```python
from build123d import *

# Parameters (mm, degrees)
BASE_FLANGE1_DEPTH             = 762
HOLE1_OUTLINE_R                = 7.14375
HOLE1_DEPTH                    = 1.4986
LPATTERN1_COUNT                = 10
LPATTERN1_PITCH                = 139.7
F_5_16_0_3125_DIAMETER_HOLE1_D = 7.9375
LPATTERN2_COUNT                = 10
LPATTERN2_PITCH                = 139.7


# Read off the part's stored shape, not the designer's step: Hole1
# Sheet-metal steps are written as plain solids
with BuildPart() as part:
    # Sketch1 → Base-Flange1 (new, symmetric)
    with BuildSketch(Plane.XY):
        with BuildLine():
            Line((82.55, 50.8), (82.55, 3.0861))
            ThreePointArc((82.55, 3.0861), (81.646102237, 0.903897763), (79.4639, 0))
            Line((79.4639, 0), (-79.4639, 0))
            ThreePointArc((-79.4639, 0), (-81.646102237, 0.903897763), (-82.55, 3.0861))
            Line((-82.55, 3.0861), (-82.55, 50.8))
            Line((-82.55, 50.8), (-81.0514, 50.8))
            Line((-81.0514, 50.8), (-81.0514, 3.0861))
            ThreePointArc((-81.0514, 3.0861), (-80.586432015, 1.963567985), (-79.4639, 1.4986))
            Line((-79.4639, 1.4986), (79.4639, 1.4986))
            ThreePointArc((79.4639, 1.4986), (80.586432015, 1.963567985), (81.0514, 3.0861))
            Line((81.0514, 3.0861), (81.0514, 50.8))
            Line((81.0514, 50.8), (82.55, 50.8))
        make_face()
    extrude(amount=BASE_FLANGE1_DEPTH, both=True)

    # Hole1 outline → Hole1 (cut)
    with BuildSketch(Plane(origin=(0, 0, 0), x_dir=(1, 0, 0), z_dir=(0, 1, 0))):
        with Locations((0, 628.65)):
            Circle(HOLE1_OUTLINE_R)
    hole1 = extrude(amount=HOLE1_DEPTH, mode=Mode.SUBTRACT)

    # LPattern1: Hole1 ×10
    with Locations(*[(0, 0, i * LPATTERN1_PITCH) for i in range(1, LPATTERN1_COUNT)]):
        add(hole1, mode=Mode.SUBTRACT)

    # 5/16 (0.3125) Diameter Hole1 (through all)
    with Locations(Plane(origin=(0, 0, 0), x_dir=(-1, 0, 0), z_dir=(0, -1, 0))):
        with Locations((0, 660.4), (0, 596.9)):
            f_5_16_0_3125_diameter_hole1 = Hole(F_5_16_0_3125_DIAMETER_HOLE1_D / 2)

    # LPattern2: 5/16 (0.3125) Diameter Hole1 ×10
    with Locations(*[(0, 0, i * LPATTERN2_PITCH) for i in range(1, LPATTERN2_COUNT)]):
        add(f_5_16_0_3125_diameter_hole1, mode=Mode.SUBTRACT)


solid = part.part
```
Read the model definition and answer for the solid it produces. Units are mm, in the model's axes. A direction names the side the tool comes from. Coordinates: 2 decimals unless noted, no trailing zeros. Order: outer loops, then holes, each group sorted by start corner. A loop starts at its lowest first (then second) coordinate and runs counter-clockwise, first axis right, second up. Notation, with made-up numbers: (2.25, 15.5) - (16.25, 15.5) arc R25 ccw to (16.25, 40.5) - close; hole circle Ø11 at (-19.5, 43). An arc over 180 degrees is marked (long way). Answer as a JSON object with one key per item and string values. Group by question number.
Item 1: The mould has two halves that part along X. Classify faces 1 (the face through (82.55, 27, 11)), 2 (the face through (81.051, 27, 11)), 3 (the face through (0, 1, 762)), 4 (the face through (-82.55, 27, 11)): +X half, -X half, draft (parallel to the pull), parting line (faces both ways), or undercut.
Item 2: Section A-A (y = 23) is taken. Give the vertices of the cut face in (x, z).
Item 3: Consider probe 1 along X at (y, z) = (26.5, 3); probe 2 along Y at (x, z) = (38, -429); probe 3 along X at (y, z) = (1.2, 520.7). Determine where each line is inside the solid, lowest interval first. Write a range as from..to.
Item 4: Flat-ended cylindrical pins translate along their axes: P1, Ø7, axis at x = 0, z = 457.2, coming from the -Y side (3 decimals); P2, Ø12.5, axis at x = 0, z = 596.9, coming from the -Y side; P3, Ø16.5, axis at x = 0, z = -628.65, coming from the +Y side. Find the tip coordinate at first contact, or state that the pin passes through.
Item 5: Section C-C (x = -48) is taken. Give the vertices of the cut face in (y, z).
Item 6: A tool of negligible diameter and unlimited length cuts with its end or side. For faces 5 (the face through (1, 0, 11)), 6 (the face through (-81.051, 27, 11)), from which of +Z, -Z, +X, -X, +Y, -Y can it reach the whole face along a straight path? Write none if from no direction.
Results are:
{
 "1": {"face 1": "+X half", "face 2": "undercut", "face 3": "draft", "face 4": "-X half"},
 "2": {"outline": "(-82.55, -762) - (-81.05, -762) - (-81.05, 762) - (-82.55, 762) - close; (81.05, -762) - (82.55, -762) - (82.55, 762) - (81.05, 762) - close"},
 "3": {"probe 1": "x = -82.55..-81.05, 81.05..82.55", "probe 2": "y = 0..1.5", "probe 3": "x = -81.91..-3.97, 3.97..81.91"},
 "4": {"P1": "passes through", "P2": "stops at y = 0", "P3": "stops at y = 1.5"},
 "5": {"outline": "(0, -762) - (1.5, -762) - (1.5, 762) - (0, 762) - close"},
 "6": {"face 5": "+Z, -Z, +X, -X, -Y", "face 6": "+Z, -Z, +Y"}
}
